Read the model definition and answer for the solid it produces. Units are mm, in the model's axes. Face numbers are marked on the shaded views. Coordinates: 2 decimals unless noted, no trailing zeros. Order: outer loops, then holes, each group sorted by start corner. A loop starts at its lowest first (then second) coordinate and runs counter-clockwise, first axis right, second up. Notation, with made-up numbers: (-24.75, 18.5) - (3.25, 18.5) arc R22 cw to (3.25, 45.5) - close; hole circle Ø11 at (-13.5, 72). An arc over 180 degrees is marked (long way). Use one line per item in the form item = value.
```python
from build123d import *

# Parameters (mm, degrees)
F0_R     = 9.525
F1_DEPTH = 19.05
F2_R     = 6.731
F3_DEPTH = 12.7
F4_R     = 1.27


with BuildPart() as f1:
    # F0 (on Top) → F1 (new body)
    with BuildSketch(Plane.XY):
        Circle(F0_R)
    extrude(amount=F1_DEPTH)

    # F2 (on face) → F3 (cut)
    with BuildSketch(Plane.XY.offset(19.05)):
        Circle(F2_R)
    extrude(amount=-F3_DEPTH, mode=Mode.SUBTRACT)

    # F4
    f4_edges = [f1.edges().sort_by_distance(p)[0] for p in [
        (-9.525, 0, 0),
    ]]
    fillet(f4_edges, radius=F4_R)


solid = f1.part
```
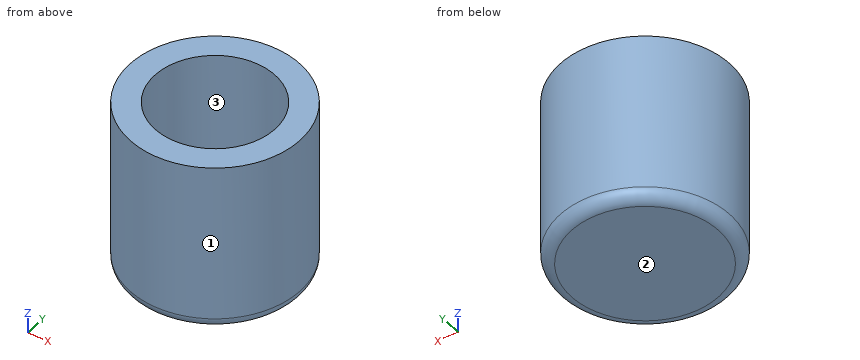
(1) The mould has two halves that part along X. Classify the marked faces 1, 2 and 3: +X half, -X half, draft (parallel to the pull), parting line (faces both ways), or undercut.
Answer list:
face_1 = parting line
face_2 = draft
face_3 = undercut
(2) Section D-D, the plane z = 6 is taken. Write down the section's boundary in (x, y) (3 decimals).
Answer list:
outline = circle Ø19.05 at (0, 0)
(3) Given pin 1 Ø2 at (y, z) = (2, 6) entering from -X; pin 2 Ø5 at (y, z) = (3.5, 7) entering from +X; pin 3 Ø2 at (x, z) = (2.5, 11.5) entering from +Y, each flat-ended and moving along its own axis, determine where each tip first touches the part or whether it passes through.
Answer list:
pin_1 = -9.47
pin_2 = 9.47
pin_3 = 9.41
(4) Section C-C, the plane z = 11 is taken. Write down the section's boundary in (x, y) (3 decimals).
Answer list:
outline = circle Ø19.05 at (0, 0); hole circle Ø13.462 at (0, 0)
(5) Straight lines are drawn through the part: L1, parallel to Y at x = 0, z = 10.75 (3 decimals); L2, parallel to Z at x = 1, y = -6.5; L3, parallel to Y at x = -2.5, z = 14. For each, find the intervals that lie inside material, in ascending order.
Answer list:
L1 = -9.525 to -6.731, 6.731 to 9.525
L2 = 0 to 6.35
L3 = -9.19 to -6.25, 6.25 to 9.19
(6) Section A-A, the plane y = 0 is taken. Write down the section's boundary in (x, z) (3 decimals).
Answer list:
outline = (-9.525, 1.27) arc R1.27 ccw to (-8.255, 0) - (8.255, 0) arc R1.27 ccw to (9.525, 1.27) - (9.525, 19.05) - (6.731, 19.05) - (6.731, 6.35) - (-6.731, 6.35) - (-6.731, 19.05) - (-9.525, 19.05) - close
